Autodesk Inventor part; units mm, degrees
ref_plane "Work Plane1" through (-27, 3, 0) normal (-0.7071, 0.7071, 0) x (0, 0, 1)
ref_plane "YZ Plane" through (0, 0, 0) normal (1, 0, 0) x (0, 1, 0)
ref_plane "XZ Plane" through (0, 0, 0) normal (0, 1, 0) x (-1, 0, 0)
sketch "Sketch1" plane through (0, 0, 0) normal (0, 1, 0) x (-1, 0, 0)
  line L0 (-30, -15) -> (30, -15)
  line L1 (30, -15) -> (30, 15)
  line L2 (30, 15) -> (-30, 15)
  line L3 (-30, 15) -> (-30, -15)
  line L4 (-30, -15) -> (30, 15) construction
  line L5 (30, -15) -> (-30, 15) construction
  point P0 (0, 0)
  dimension "d0" = 60
  dimension "d1" = 30
extrude "Extrusion1" add sketch "Sketch1" along normal blind 3
sketch "Sketch2" plane through (0, 3, 0) normal (0, 1, 0) x (1, 0, 0)
  line L0 (-30, 15) -> (-30, -15)
  line L1 (30, 15) -> (-30, 15)
  line L2 (-30, -15) -> (-27, -15)
  line L3 (-27, -15) -> (-27, 15)
  line L4 (-27, 15) -> (-30, 15)
  line L5 (-30, 15) -> (-30, -15)
  point P0 (0, 0)
  dimension "d4" = 3
extrude "Extrusion2" add sketch "Sketch2" along normal blind 57
sketch "Sketch3" plane through (0, 3, 0) normal (0, 1, 0) x (1, 0, 0)
  line L0 (-7, 0) -> (13, 0) construction
  line L1 (-7, -5) -> (13, -5)
  line L2 (13, 5) -> (-7, 5)
  arc A0 (-7, 5) -> (-7, -5) centre (-7, 0) ccw
  arc A1 (13, -5) -> (13, 5) centre (13, 0) ccw
  line L3 (3, 0) -> (23, 0) construction
  line L4 (-27, -15) -> (30, -15)
  line L5 (30, -15) -> (30, 15)
  circle A2 centre (18, -10) radius 2.5
  point P0 (18, 0)
  dimension "d7" = 10
  dimension "d8" = 0
  dimension "d9" = 10
  dimension "d10" = 5
  dimension "d11" = 12
  dimension "d12" = 5
  dimension "d23" = 0
extrude "Extrusion3" cut sketch "Sketch3" against normal through all contours A2
pattern_linear "Rectangular Pattern1" count 2 spacing 30 along (-1, 0, 0) count 2 spacing 20 along (0, 0, -1) of "Extrusion3"
extrude "Extrusion4" cut sketch "Sketch3" against normal through all contours A0 L2 A1 L1
ref_plane "Work Plane1" through (-27, 3, 0) normal (-0.7071, 0.7071, 0) x (0, 0, 1)
mirror "Mirror1" about plane through (-27, 3, 0) normal (-0.7071, 0.7071, 0) of "Extrusion3", "Rectangular Pattern1", "Extrusion4"
properties part number "L_Bracket"
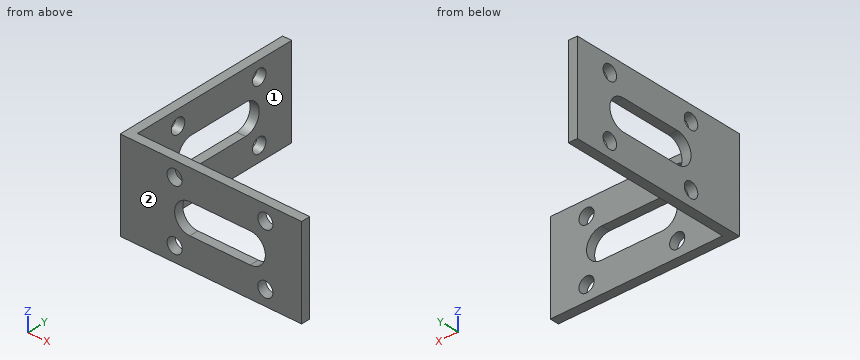
Here's how the part is built. I have some questions about the finished solid (model axes, mm). Face numbers are marked on the shaded views. A direction names the side the tool comes from. Round coordinates to 2 decimals unless told otherwise and drop trailing zeros. Loops run counter-clockwise (first coordinate to the right, second up) from the corner with the lowest first, then second, coordinate; pieces in that order, holes last. Notation, with made-up numbers: (-37, -1.75) - (19, -1.75) arc R12 ccw to (19, 18.25) - close; hole circle Ø1 at (-29, 30.25). An arc over 180 degrees is marked (long way). One line per question, with ' | ' between items. Start each with the question number.
Q1. I want a section at D-D (x = 19). Write out the boundary of the cut face in (y, z).
Q2. Please list where these lines run through material, in increasing order: line 1 (Y direction, x = -28.8, z = 10); line 2 (X direction, y = 1.3, z = 10); line 3 (Y direction, x = -13, z = 12.5). Write a range as [from, to].
Q3. I want a section at A-A (y = 24). Write out the boundary of the cut face in (x, z).
Q4. I want a section at B-B (x = 1). Write out the boundary of the cut face in (y, z), then the cut area to 3 significant figures.
Q5. For the marked faces 1 and 2, which set-ups out of +Z, -Z, +X, -X, +Y, -Y let a thin tool reach every point of the face, with its end or its side?
Q6. I want a section at C-C (z = -3.75). Write out the boundary of the cut face in (x, y), then the cut area to 3 significant figures.
Q7. Will these pins go through, and if not, where does the flat tip stop? pin 1 (6 mm diameter, centred on x = 9.5, z = 5, fed in from +Y); pin 2 (2 mm diameter, centred on x = 0.5, z = 3.5, fed in from -Y); pin 3 (6 mm diameter, centred on y = 18, z = -10, fed in from +X).
Response values:
1) outline: (0, -15) - (3, -15) - (3, -12.29) - (0, -12.29) - close; (0, -7.71) - (3, -7.71) - (3, 7.71) - (0, 7.71) - close; (0, 12.29) - (3, 12.29) - (3, 15) - (0, 15) - close
2) line 1: y = [0, 15.5], [20.5, 45.5], [50.5, 60] | line 2: x = [-30, -14.5], [-9.5, 15.5], [20.5, 30] | line 3: y = [0, 3]
3) outline: (-30, -15) - (-27, -15) - (-27, -5) - (-30, -5) - close; (-30, 5) - (-27, 5) - (-27, 15) - (-30, 15) - close
4) outline: (0, -15) - (3, -15) - (3, -5) - (0, -5) - close; (0, 5) - (3, 5) - (3, 15) - (0, 15) - close | area: 60.0 mm²
5) face 1: +Z, -Z, +X, +Y | face 2: +Z, -Z, +X, -X, -Y
6) outline: (-30, 0) - (-10.31, 0) - (-10.31, 3) - (-27, 3) - (-27, 19.69) - (-30, 19.69) - close; (-30, 46.31) - (-27, 46.31) - (-27, 60) - (-30, 60) - close; (16.31, 0) - (30, 0) - (30, 3) - (16.31, 3) - close | area: 191 mm²
7) pin 1: stops at y = 3 | pin 2: passes through | pin 3: stops at x = -27
